Source: CAD feature listing. Evaluate the final solid. Frame: model axes, mm. Give positions to 0.01 mm unless a question says otherwise; leave off trailing zeros. Order: outer loops, then holes, each group sorted by start corner. A loop starts at its lowest first (then second) coordinate and runs counter-clockwise, first axis right, second up. Notation, with made-up numbers: M 87,35.25 L 125,35.25 A10 cw 125,53.25 Z; hole C -3.5,60.5 d6. An arc over 180 degrees is marked long. Answer in a Markdown table with one row per item. Add a question column.
(1) Section query A-A, the plane y = 2.25. Return loops of the section in (x, z).
(2) Material intervals for line 1 along Z through (x, y) = (70, 2.1); line 2 along X through (y, z) = (1, 0); line 3 along X through (y, z) = (4.2, -84), sorted ascending.
(3) Pin query (flat end, axial travel): P1, Ø1.5, axis at x = -149, y = 2, coming from the -Z side; P2, Ø1.5, axis at x = 150.5, y = 3.5, coming from the +Z side; P3, Ø2.5, axis at y = 2, z = 154, coming from the +X side. Return the tip coordinate at first contact, or that it passes through.
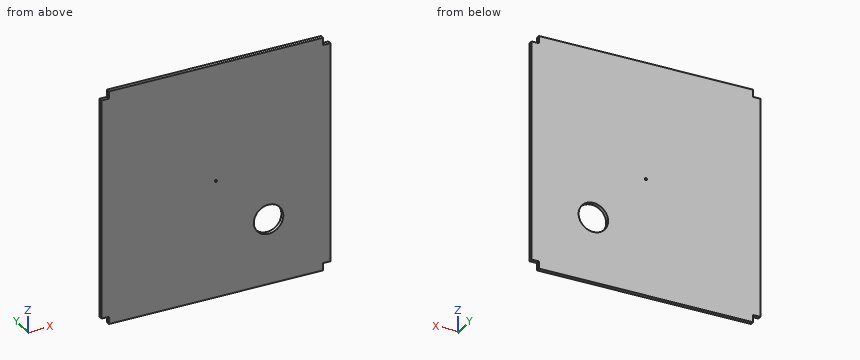
from build123d import *

# Parameters (mm, degrees)
SKETCH_1_W          = 310
SKETCH_1_H          = 320
EXTRUDE_1_DEPTH     = 5
SKETCH_4_R          = 1.5
SKETCH_4_R_2        = 20
SKETCH_4_W          = 10
SKETCH_4_H          = 10
CUT_EXTRUDE_2_DEPTH = 5


with BuildPart() as part:
    # 草图1 → 凸台-拉伸1 (new body)
    with BuildSketch(Plane(origin=(0, 0, 0), x_dir=(1, 0, 0), z_dir=(0, 1, 0))):
        Rectangle(SKETCH_1_W, SKETCH_1_H)
    extrude(amount=EXTRUDE_1_DEPTH)

    # 草图4 → 切除-拉伸2 (cut)
    with BuildSketch(Plane(origin=(0, 5, 0), x_dir=(1, 0, 0), z_dir=(0, 1, 0))):
        with Locations(Location((0, 0, 0), (0, 0, 270))):
            Circle(SKETCH_4_R)
        with Locations(Location((71.315589165, 70.826615801, 0), (0, 0, 270))):
            Circle(SKETCH_4_R_2)
        with Locations((-150, 155)):
            Rectangle(SKETCH_4_W, SKETCH_4_H)
        with Locations((-150, -155)):
            Rectangle(SKETCH_4_W, SKETCH_4_H)
        with Locations((150, -155)):
            Rectangle(SKETCH_4_W, SKETCH_4_H)
        with Locations((150, 155)):
            Rectangle(SKETCH_4_W, SKETCH_4_H)
    extrude(amount=-CUT_EXTRUDE_2_DEPTH, mode=Mode.SUBTRACT)


solid = part.part
Values follow:
| question | item | result |
|---|---|---|
| 1 | outline | M -155,-150 L -145,-150 L -145,-160 L 145,-160 L 145,-150 L 155,-150 L 155,150 L 145,150 L 145,160 L -145,160 L -145,150 L -155,150 Z; hole C 0,0 d3; hole C 71.32,-70.83 d40 |
| 2 | line 1 | z = -160 to -90.78, -50.87 to 160 |
| 2 | line 2 | x = -155 to -1.5, 1.5 to 155 |
| 2 | line 3 | x = -155 to 56.27, 86.36 to 155 |
| 3 | P1 | stops at z = -150 |
| 3 | P2 | stops at z = 150 |
| 3 | P3 | stops at x = 145 |
